Here's the drawing with two shaded views (mm, measured from the low corner). I have some questions. A direction names the side the tool comes from. Coordinates: 2 decimals unless noted, no trailing zeros. Write each loop counter-clockwise with the first axis right and the second up, starting at its lowest first coordinate (ties: lowest second). Pieces come first, ordered by that corner, then holes.
Item 1: If I drill on probe 1 along Y at (x, z) = (12, 6.5); probe 2 along Z at (x, y) = (20, 34.5); probe 3 along X at (y, z) = (8.5, 9.75), over which ranges is the centre line in solid material (lowest first)?
Item 2: For P1, Ø5, axis at x = 23, z = 9, coming from the +Y side; P2, Ø5, axis at y = 17.5, z = 7, coming from the +X side; P3, Ø5, axis at y = 4.5, z = 8.5, coming from the +X side, each with a flat end and sliding along its axis, tell me the tip position at first contact or that it passes through.
Item 3: I want a section at B-B on x = 19. Please give me the cut outline in (y, z), then the cut area to 3 significant figures.
Item 4: I want a section at D-D on y = 15. Please give me the cut outline in (x, z), then the cut area to 3 significant figures.
Item 5: I want a section at C-C on y = 29. Please give me the cut outline in (x, z).
Item 6: Thinking about a two-plate mould opening in X: for the marked faces 4, 5 and 6, which applies, +X half, -X half, draft (parallel to the pull), parting line (faces both ways), or undercut?
Item 7: Which directions (+Z, -Z, +X, -X, +Y, -Y) give clear straight access to the entire face, cutting with the end or side of a thin tool? Please do the marked faces 1, 2 and 3.
Item 8: I want a section at A-A on z = 4. Please give me the cut outline in (x, y).
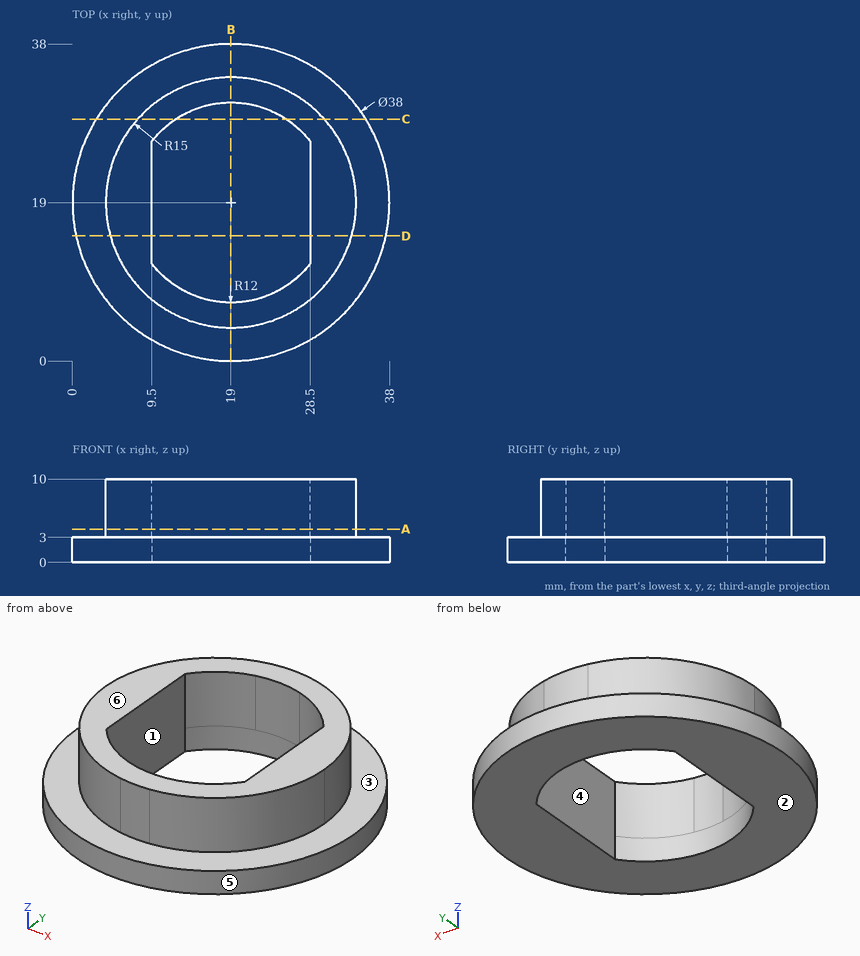
Response values:
1. probe 1: y = 5.73 to 9.25, 28.75 to 32.27
1. probe 2: z = 0 to 3
1. probe 3: x = 8.29 to 13.19, 24.81 to 29.71
2. P1: stops at y = 33.92
2. P2: stops at x = 34
2. P3: stops at x = 28
3. outline: (0, 0) - (7, 0) - (7, 10) - (4, 10) - (4, 3) - (0, 3) - close; (31, 0) - (38, 0) - (38, 3) - (34, 3) - (34, 10) - (31, 10) - close
3. area: 84.0 mm2
4. outline: (0.43, 0) - (9.5, 0) - (9.5, 10) - (4.54, 10) - (4.54, 3) - (0.43, 3) - close; (28.5, 0) - (37.57, 0) - (37.57, 3) - (33.46, 3) - (33.46, 10) - (28.5, 10) - close
4. area: 124 mm2
5. outline: (2.84, 0) - (12.37, 0) - (12.37, 10) - (7.82, 10) - (7.82, 3) - (2.84, 3) - close; (25.63, 0) - (35.16, 0) - (35.16, 3) - (30.18, 3) - (30.18, 10) - (25.63, 10) - close
6. face 4: undercut
6. face 5: parting line
6. face 6: draft
7. face 1: +Z, -Z
7. face 2: -Z, +X, -X, +Y, -Y
7. face 3: +Z
8. outline: circle Ø30 at (19, 19); hole (9.5, 11.67) arc R12 ccw to (28.5, 11.67) - (28.5, 26.33) arc R12 ccw to (9.5, 26.33) - close
